Autodesk Inventor part; units mm, degrees
ref_plane "YZ Plane" through (0, 0, 0) normal (1, 0, 0) x (0, 1, 0)
ref_plane "XZ Plane" through (0, 0, 0) normal (0, 1, 0) x (-1, 0, 0)
ref_plane "XY Plane" through (0, 0, 0) normal (0, 0, 1) x (1, 0, 0)
sketch "Boceto1" plane through (0, 0, 0) normal (0, 0, 1) x (1, 0, 0)
  circle A0 centre (0, 0) radius 7.94
  dimension "d0" = 15.88
extrude "Extrusión1" add sketch "Boceto1" along normal blind 53.74
sketch "Boceto4" plane through (0, 0, 0) normal (0, 0, -1) x (-1, 0, 0)
  circle A0 centre (0, 0) radius 1.7349
sketch "Boceto5" plane through (0, 0, 53.74) normal (0, 0, 1) x (1, 0, 0)
  circle A0 centre (0, 0) radius 2.5
  dimension "d17" = 5
hole "Agujero1" at (0, 0, 0) direction (0, 0, 1) diameter 5 depth 10 tip angle 118
hole "Agujero2" at (0, 0, 53.74) direction (0, 0, -1) diameter 5 depth 10 tip angle 118
thread "Rosca5"
thread "Rosca6"
properties part number "Barras_Soporte_superior" material "Acero inoxidable"
Geometry: final body of the model. Coordinates: model frame, mm. A direction names the side the tool comes from. Coordinates: 2 decimals unless noted, no trailing zeros. Order: outer loops, then holes, each group sorted by start corner. A loop starts at its lowest first (then second) coordinate and runs counter-clockwise, first axis right, second up. Notation, with made-up numbers: (-38, 28.25) - (14, 28.25) arc R16 cw to (14, 56.25) - close; hole circle Ø5 at (66, 5.5). An arc over 180 degrees is marked (long way). Return JSON: item names as keys, results as strings. Group by question number.
1. Pull-direction query (X, two-part tool) for faces 1 (the face through (2, 2, 0)), 2 (the face through (2.44, -0.54, 5.07)), 3 (the face through (7.573, -2.385, 26.494)), 4 (the face through (-0.424, -0.094, 11.241)); classes: pulls with the +X half, pulls with the -X half, needs draft (parallel to the pull), parting line crosses it, or undercut.
2. Cut plane A-A (z = 7). Output: boundary loops of the cut face in (x, y).
3. Cut plane D-D (z = 23.5). Output: boundary loops of the cut face in (x, y).
4. Cut plane C-C (x = 4.5). Output: boundary loops of the cut face in (y, z).
5. Cut plane B-B (y = 6.5). Output: boundary loops of the cut face in (x, z).
6. Material intervals for line 1 along Y through (x, z) = (0, 48.25); line 2 along Y through (x, z) = (-0.75, 7.5); line 3 along X through (y, z) = (2, 36), sorted ascending. Write a range as [from, to].
7. Set-up query: faces 5 (the face through (2.44, 0.54, 48.67)), 6 (the face through (2, 2, 53.74)). Return all of +Z, -Z, +X, -X, +Y, -Y with unobstructed straight access to the full face (end or side cutting, diameter ignored); none if empty.
8. Pin query (flat end, axial travel): pin 1 (3 mm diameter, centred on x = 0, y = 0, fed in from +Z); pin 2 (5 mm diameter, centred on x = 1, z = 10.5, fed in from +Y); pin 3 (3 mm diameter, centred on x = 4.5, z = 32, fed in from +Y); pin 4 (4.5 mm diameter, centred on x = 0, y = 0, fed in from -Z). Return the tip coordinate at first contact, or that it passes through.
Resolved:
{
 "1": {"face 1": "needs draft", "face 2": "undercut", "face 3": "parting line crosses it", "face 4": "undercut"},
 "2": {"outline": "circle Ø15.88 at (0, 0); hole circle Ø5 at (0, 0)"},
 "3": {"outline": "circle Ø15.88 at (0, 0)"},
 "4": {"outline": "(-6.54, 0) - (6.54, 0) - (6.54, 53.74) - (-6.54, 53.74) - close"},
 "5": {"outline": "(-4.56, 0) - (4.56, 0) - (4.56, 53.74) - (-4.56, 53.74) - close"},
 "6": {"line 1": "y = [-7.94, -2.5], [2.5, 7.94]", "line 2": "y = [-7.9, -2.38], [2.38, 7.9]", "line 3": "x = [-7.68, 7.68]"},
 "7": {"face 5": "+Z", "face 6": "+Z, +X, -X, +Y, -Y"},
 "8": {"pin 1": "stops at z = 43.14", "pin 2": "stops at y = 7.94", "pin 3": "stops at y = 7.35", "pin 4": "stops at z = 10.15"}
}
